from build123d import *

# Parameters (mm, degrees)
F0_R     = 16.125
F0_R_2   = 9.445
F1_DEPTH = 22.67
F0_R_3   = 7.02
F3_DEPTH = 20.53
F0_R_4   = 4.02
F5_DEPTH = 13
F6_DEPTH = 6.5
F7_DEPTH = 11.3


with BuildPart() as f1:
    # F0 (on Front) → F1 (new body)
    with BuildSketch(Plane.XZ):
        Circle(F0_R)
        Circle(F0_R_2, mode=Mode.SUBTRACT)
    extrude(amount=F1_DEPTH)

    # F0 (on Front) → F3 (join)
    with BuildSketch(Plane.XZ):
        Circle(F0_R_2)
        Circle(F0_R_3, mode=Mode.SUBTRACT)
    extrude(amount=F3_DEPTH)

    # F0 (on Front) → F5 (join)
    with BuildSketch(Plane.XZ):
        Circle(F0_R_3)
        Circle(F0_R_4, mode=Mode.SUBTRACT)
    extrude(amount=F5_DEPTH)

    # F0 (on Front) → F6 (join)
    with BuildSketch(Plane.XZ):
        Circle(F0_R_4)
        with BuildLine():
            ThreePointArc((2.971368, 1.06066), (3.108753, 0.538219), (3.155, 0))
            ThreePointArc((3.155, 0), (3.108753, -0.538219), (2.971368, -1.06066))
            ThreePointArc((2.971368, -1.06066), (0, -3.155), (-2.971368, -1.06066))
            ThreePointArc((-2.971368, -1.06066), (-3.155, 0), (-2.971368, 1.06066))
            ThreePointArc((-2.971368, 1.06066), (0, 3.155), (2.971368, 1.06066))
        make_face(mode=Mode.SUBTRACT)
    extrude(amount=F6_DEPTH)

    # F0 (on Front) → F7 (join)
    with BuildSketch(Plane.XZ):
        Circle(F0_R)
        Circle(F0_R_2, mode=Mode.SUBTRACT)
        with BuildLine():
            Line((-1.910707, 0), (-2.971368, 1.06066))
            ThreePointArc((-2.971368, 1.06066), (-3.155, 0), (-2.971368, -1.06066))
            Line((-2.971368, -1.06066), (-1.910707, 0))
        make_face()
        with BuildLine():
            ThreePointArc((2.971368, -1.06066), (3.108753, -0.538219), (3.155, 0))
            ThreePointArc((3.155, 0), (3.108753, 0.538219), (2.971368, 1.06066))
            Line((2.971368, 1.06066), (1.910707, 0))
            Line((1.910707, 0), (2.971368, -1.06066))
        make_face()
    extrude(amount=F7_DEPTH)


solid = f1.part
The listing builds one solid part. Answer for the finished solid, in the listing's coordinates (mm). A direction names the side the tool comes from. Round coordinates to 2 decimals unless told otherwise and drop trailing zeros. Loops run counter-clockwise (first coordinate to the right, second up) from the corner with the lowest first, then second, coordinate; pieces in that order, holes last. Notation, with made-up numbers: M 69,79.5 L 108,79.5 A6 cw 108,84.5 Z; hole C 11.25,29.25 d8. An arc over 180 degrees is marked long. Write each question's results on one line, items separated by ' | '. Start each with the question number.
1) Determine the mould class of faces 4 (the flat face through (-1.44, -20.53, 7.04)), 5 (the cylindrical face through (15.38, -11.18, 4.84)), 6 (the flat face through (7, -22.67, -7)) for opening direction Z: pulls with the +Z half, pulls with the -Z half, needs draft (parallel to the pull), parting line crosses it, or undercut.
2) Straight lines are drawn through the part: probe 1 along Z at (x, y) = (0, -8.5) (3 decimals); probe 2 along Z at (x, y) = (0, -22.1) (3 decimals); probe 3 along Y at (x, z) = (7.5, 3). For each, find the intervals that lie inside material, in ascending order.
3) Find section A-A on x = 0. Write down the section's boundary in (y, z) (3 decimals).
4) Find section C-C on y = -4.75. Write down the section's boundary in (x, z) (3 decimals), plus the area to 3 significant figures.
5) Find section B-B on y = -7.75. Write down the section's boundary in (x, z) (3 decimals).
6) Each of these flat-tipped pins is pushed along its axis until it touches: pin 1 (4 mm diameter, centred on x = -1, z = 1.5, fed in from -Y); pin 2 (2 mm diameter, centred on y = -8.5, z = -9, fed in from -X); pin 3 (2.5 mm diameter, centred on x = 1.5, z = 1.5, fed in from -Y). Where does it stop, or does it pass through?
7) Which of the six approach directions +Z, -Z, +X, -X, +Y, -Y give full straight-line access (tool end or side, diameter ignored) to faces 1 (the flat face through (3, 0, 0)), 2 (the flat face through (2.45, -5.57, 0.54)), 3 (the cylindrical face through (-1.23, -21.585, 9.365))?
8) Find section D-D on z = -2.5. Write down the section's boundary in (x, y), plus the area to 3 significant figures.
Final values:
1) face 4: undercut | face 5: parting line crosses it | face 6: needs draft
2) probe 1: -16.125 to -4.02, 4.02 to 16.125 | probe 2: -16.125 to -9.445, 9.445 to 16.125 | probe 3: -20.53 to 0
3) outline: M -22.67,-16.125 L 0,-16.125 L 0,-3.155 L -6.5,-3.155 L -6.5,-4.02 L -13,-4.02 L -13,-7.02 L -20.53,-7.02 L -20.53,-9.445 L -22.67,-9.445 Z; M -22.67,9.445 L -20.53,9.445 L -20.53,7.02 L -13,7.02 L -13,4.02 L -6.5,4.02 L -6.5,3.155 L 0,3.155 L 0,16.125 L -22.67,16.125 Z
4) outline: C 0,0 d32.25; hole M -2.971,-1.061 A3.155 ccw 2.971,-1.061 L 1.911,0 L 2.971,1.061 A3.155 ccw -2.971,1.061 L -1.911,0 Z | area: 788 mm²
5) outline: C 0,0 d32.25; M -2.971,-1.061 L -1.911,0 L -2.971,1.061 A3.155 ccw Z; M 1.911,0 L 2.971,-1.061 A3.155 ccw 3.155,0 A3.155 ccw 2.971,1.061 Z; hole C 0,0 d8.04
6) pin 1: y = -11.3 | pin 2: x = -14 | pin 3: y = -6.5
7) face 1: +Z, -Z, +X, -X, +Y | face 2: +Y, -Y | face 3: -Y
8) outline: M -15.93,-22.67 L -9.11,-22.67 L -9.11,-20.53 L -6.56,-20.53 L -6.56,-13 L -3.15,-13 L -3.15,-6.5 L -1.92,-6.5 L -1.92,0 L -15.93,0 Z; M 1.92,-6.5 L 3.15,-6.5 L 3.15,-13 L 6.56,-13 L 6.56,-20.53 L 9.11,-20.53 L 9.11,-22.67 L 15.93,-22.67 L 15.93,0 L 1.92,0 Z | area: 519 mm²
